Design review of the part built by this model. Coordinates are the model's own, in mm. Face numbers are marked on the shaded views. A direction names the side the tool comes from. Coordinates: 2 decimals unless noted, no trailing zeros. Loops run counter-clockwise (first coordinate to the right, second up) from the corner with the lowest first, then second, coordinate; pieces in that order, holes last. Notation, with made-up numbers: (50.25, 63.25) -> (96.25, 63.25) arc R32 ccw to (96.25, 100.25) -> close; hole circle Ø5 at (44, 62). An arc over 180 degrees is marked (long way). Answer as a JSON object with one key per item and string values.
```python
from build123d import *

# Parameters (mm, degrees)
BOSS_EXTRUDE1_DEPTH     = 17.5
CUT_EXTRUDE1_REACH      = 28.315
CUT_EXTRUDE1_END_RADIUS = 8.05
SKETCH2_R               = 1.55


with BuildPart() as part:
    # Sketch1 → Boss-Extrude1 (new, symmetric)
    with BuildSketch(Plane.XY):
        with BuildLine():
            Line((-11.27, 11.27), (11.27, 11.27))
            Line((11.27, 11.27), (11.27, -4.83))
            Line((11.27, -4.83), (8.05, -4.83))
            Line((8.05, -4.83), (8.05, 0))
            ThreePointArc((8.05, 0), (0, 8.05), (-8.05, 0))
            Line((-8.05, 0), (-8.05, -4.83))
            Line((-8.05, -4.83), (-11.27, -4.83))
            Line((-11.27, -4.83), (-11.27, 11.27))
        make_face()
    extrude(amount=BOSS_EXTRUDE1_DEPTH, both=True)

    # Cut-Extrude1: up to this cylinder (the profile starts outside it)
    cut_extrude1_end = Plane(origin=(0, 0, -4.5), z_dir=(0, 0, -1)) * Cylinder(CUT_EXTRUDE1_END_RADIUS, 83.73, mode=Mode.PRIVATE)
    # Sketch2 → Cut-Extrude1 (cut, up to the surface)
    with BuildSketch(Plane(origin=(0, 11.27, 0), x_dir=(1, 0, 0), z_dir=(0, 1, 0)), mode=Mode.PRIVATE) as cut_extrude1_sk1:
        with Locations(Location((0, 9.5, 0), (0, 0, 270))):
            Circle(SKETCH2_R)
    cut_extrude1_tool1 = extrude(cut_extrude1_sk1.sketch, amount=-CUT_EXTRUDE1_REACH, mode=Mode.PRIVATE) - cut_extrude1_end
    add(cut_extrude1_tool1.solids().sort_by_distance((0, 11.27, -9.5))[0], mode=Mode.SUBTRACT)
    # Sketch2 → Cut-Extrude1 (cut, up to the surface)
    with BuildSketch(Plane(origin=(0, 11.27, 0), x_dir=(1, 0, 0), z_dir=(0, 1, 0)), mode=Mode.PRIVATE) as cut_extrude1_sk2:
        with Locations(Location((0, -0.5, 0), (0, 0, 270))):
            Circle(SKETCH2_R)
    cut_extrude1_tool2 = extrude(cut_extrude1_sk2.sketch, amount=-CUT_EXTRUDE1_REACH, mode=Mode.PRIVATE) - cut_extrude1_end
    add(cut_extrude1_tool2.solids().sort_by_distance((0, 11.27, 0.5))[0], mode=Mode.SUBTRACT)


solid = part.part
```
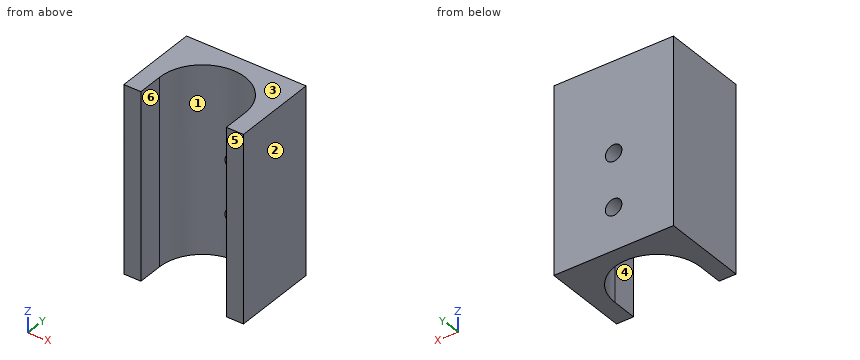
1) Add section D-D, the plane y = 9.75. Give the boundary of the cut face in (x, z).
Completed:
{"outline": "(-11.27, -17.5) -> (11.27, -17.5) -> (11.27, 17.5) -> (-11.27, 17.5) -> close; hole circle Ø3.1 at (0, -9.5); hole circle Ø3.1 at (0, 0.5)"}
2) Add section A-A, the plane x = 0. Give the boundary of the cut face in (y, z), and give its area (3 significant figures).
Completed:
{"outline": "(8.05, -17.5) -> (11.27, -17.5) -> (11.27, -11.05) -> (8.05, -11.05) -> close; (8.05, -7.95) -> (11.27, -7.95) -> (11.27, -1.05) -> (8.05, -1.05) -> close; (8.05, 2.05) -> (11.27, 2.05) -> (11.27, 17.5) -> (8.05, 17.5) -> close", "area": "92.7 mm²"}
3) Wall thickness on probe 1 along Z at (x, y) = (0, 10.2); probe 2 along X at (y, z) = (-1.25, -9); probe 3 along X at (y, z) = (9.2, -9.5): over which ranges is each line inside the solid? List them lowest first.
Completed:
{"probe 1": "-17.5 to -11.05, -7.95 to -1.05, 2.05 to 17.5", "probe 2": "-11.27 to -8.05, 8.05 to 11.27", "probe 3": "-11.27 to -1.55, 1.55 to 11.27"}
4) Add section B-B, the plane y = -0.75. Give the boundary of the cut face in (x, z), and give its area (3 significant figures).
Completed:
{"outline": "(-11.27, -17.5) -> (-8.05, -17.5) -> (-8.05, 17.5) -> (-11.27, 17.5) -> close; (8.05, -17.5) -> (11.27, -17.5) -> (11.27, 17.5) -> (8.05, 17.5) -> close", "area": "225 mm²"}
5) Clearance check with a flat-ended pin moving along its axis: pin 1 Ø2.5 at (x, z) = (0, 0.5) entering from -Y. State where the tip first meets the part, or that it passes through.
Completed:
{"pin 1": "through"}
6) Add section C-C, the plane z = -9.5. Give the boundary of the cut face in (x, y).
Completed:
{"outline": "(-11.27, -4.83) -> (-8.05, -4.83) -> (-8.05, 0) arc R8.05 cw to (-1.55, 7.9) -> (-1.55, 11.27) -> (-11.27, 11.27) -> close; (1.55, 7.9) arc R8.05 cw to (8.05, 0) -> (8.05, -4.83) -> (11.27, -4.83) -> (11.27, 11.27) -> (1.55, 11.27) -> close"}
7) The part is to be moulded in two halves that separate along X. For the marked faces 1, 2, 3 and 4, say which applies: pulls with the +X half, pulls with the -X half, needs draft (parallel to the pull), parting line crosses it, or undercut.
Completed:
{"face 1": "undercut", "face 2": "pulls with the +X half", "face 3": "needs draft", "face 4": "undercut"}
8) For the marked faces 5 and 6, list the 3-axis set-ups (+Z, -Z, +X, -X, +Y, -Y) from which the entire face can be reached by the end or side of a thin tool; tool diameter is ignored.
Completed:
{"face 5": "+Z, -Z, +X, -X, -Y", "face 6": "+Z, -Z, -Y"}
